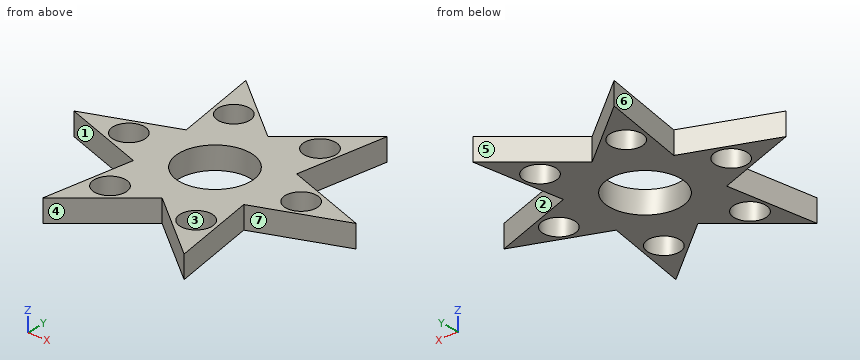
```python
from build123d import *

# Parameters (mm, degrees)
F0_R     = 4.9
F0_R_2   = 11.15
F1_DEPTH = 7


with BuildPart() as f1:
    # F0 (on Top) → F1 (new body)
    with BuildSketch(Plane.XY):
        Polygon((-7.7780097821, 13.4719081244), (0, 19.9143218109), (-22.0348406583, 38.1654635569), (-17.2463085873, 9.9571609054), align=None)
        with Locations((-13.4494397789, 23.2951130304)):
            Circle(F0_R, mode=Mode.SUBTRACT)
        with BuildLine():
            ThreePointArc((-6.4179147594, 13.9767918736), (0, 15.3798680403), (6.4179147594, 13.9767918736))
            Line((6.4179147594, 13.9767918736), (7.7780097821, 13.4719081244))
            Line((7.7780097821, 13.4719081244), (0, 19.9143218109))
            Line((0, 19.9143218109), (-7.7780097821, 13.4719081244))
            Line((-7.7780097821, 13.4719081244), (-6.4179147594, 13.9767918736))
        make_face()
        Polygon((0, 19.9143218109), (7.7780097821, 13.4719081244), (17.2463085873, 9.9571609054), (22.0348406583, 38.1654635569), align=None)
        with Locations((13.4494397789, 23.2951130304)):
            Circle(F0_R, mode=Mode.SUBTRACT)
        with BuildLine():
            ThreePointArc((8.8952994462, 12.5464731577), (13.3193564297, 7.6899340201), (15.3132142056, 1.4303187159))
            Line((15.3132142056, 1.4303187159), (15.5560195643, 0))
            Line((15.5560195643, 0), (17.2463085873, 9.9571609054))
            Line((17.2463085873, 9.9571609054), (7.7780097821, 13.4719081244))
            Line((7.7780097821, 13.4719081244), (8.8952994462, 12.5464731577))
        make_face()
        Polygon((17.2463085873, 9.9571609054), (15.5560195643, 0), (17.2463085873, -9.9571609054), (44.0696813166, 0), align=None)
        with Locations((26.8988795578, 0)):
            Circle(F0_R, mode=Mode.SUBTRACT)
        with BuildLine():
            ThreePointArc((15.3132142056, -1.4303187159), (15.3631955447, -0.7159354654), (15.3798680403, 0))
            ThreePointArc((15.3798680403, 0), (15.3631955447, 0.7159354654), (15.3132142056, 1.4303187159))
            ThreePointArc((15.3132142056, 1.4303187159), (13.3193564297, 7.6899340201), (8.8952994462, 12.5464731577))
            ThreePointArc((8.8952994462, 12.5464731577), (7.6899340201, 13.3193564297), (6.4179147594, 13.9767918736))
            ThreePointArc((6.4179147594, 13.9767918736), (0, 15.3798680403), (-6.4179147594, 13.9767918736))
            ThreePointArc((-6.4179147594, 13.9767918736), (-7.6899340201, 13.3193564297), (-8.8952994462, 12.5464731577))
            ThreePointArc((-8.8952994462, 12.5464731577), (-13.3193564297, 7.6899340201), (-15.3132142056, 1.4303187159))
            ThreePointArc((-15.3132142056, 1.4303187159), (-15.3798680403, 0), (-15.3132142056, -1.4303187159))
            ThreePointArc((-15.3132142056, -1.4303187159), (-13.3193564297, -7.6899340201), (-8.8952994462, -12.5464731577))
            ThreePointArc((-8.8952994462, -12.5464731577), (-7.6899340201, -13.3193564297), (-6.4179147594, -13.9767918736))
            ThreePointArc((-6.4179147594, -13.9767918736), (0, -15.3798680403), (6.4179147594, -13.9767918736))
            ThreePointArc((6.4179147594, -13.9767918736), (7.6899340201, -13.3193564297), (8.8952994462, -12.5464731577))
            ThreePointArc((8.8952994462, -12.5464731577), (13.3193564297, -7.6899340201), (15.3132142056, -1.4303187159))
        make_face()
        Circle(F0_R_2, mode=Mode.SUBTRACT)
        with BuildLine():
            Line((15.5560195643, 0), (15.3132142056, -1.4303187159))
            ThreePointArc((15.3132142056, -1.4303187159), (13.3193564297, -7.6899340201), (8.8952994462, -12.5464731577))
            Line((8.8952994462, -12.5464731577), (7.7780097821, -13.4719081244))
            Line((7.7780097821, -13.4719081244), (17.2463085873, -9.9571609054))
            Line((17.2463085873, -9.9571609054), (15.5560195643, 0))
        make_face()
        Polygon((22.0348406583, -38.1654635569), (17.2463085873, -9.9571609054), (7.7780097821, -13.4719081244), (0, -19.9143218109), align=None)
        with Locations((13.4494397789, -23.2951130304)):
            Circle(F0_R, mode=Mode.SUBTRACT)
        with BuildLine():
            Line((7.7780097821, -13.4719081244), (6.4179147594, -13.9767918736))
            ThreePointArc((6.4179147594, -13.9767918736), (0, -15.3798680403), (-6.4179147594, -13.9767918736))
            Line((-6.4179147594, -13.9767918736), (-7.7780097821, -13.4719081244))
            Line((-7.7780097821, -13.4719081244), (0, -19.9143218109))
            Line((0, -19.9143218109), (7.7780097821, -13.4719081244))
        make_face()
        Polygon((-22.0348406583, -38.1654635569), (0, -19.9143218109), (-7.7780097821, -13.4719081244), (-17.2463085873, -9.9571609054), align=None)
        with Locations((-13.4494397789, -23.2951130304)):
            Circle(F0_R, mode=Mode.SUBTRACT)
        with BuildLine():
            Line((-7.7780097821, -13.4719081244), (-8.8952994462, -12.5464731577))
            ThreePointArc((-8.8952994462, -12.5464731577), (-13.3193564297, -7.6899340201), (-15.3132142056, -1.4303187159))
            Line((-15.3132142056, -1.4303187159), (-15.5560195643, 0))
            Line((-15.5560195643, 0), (-17.2463085873, -9.9571609054))
            Line((-17.2463085873, -9.9571609054), (-7.7780097821, -13.4719081244))
        make_face()
        Polygon((-15.5560195643, 0), (-17.2463085873, 9.9571609054), (-44.0696813166, 0), (-17.2463085873, -9.9571609054), align=None)
        with Locations((-26.8988795578, 0)):
            Circle(F0_R, mode=Mode.SUBTRACT)
        with BuildLine():
            ThreePointArc((-15.3132142056, 1.4303187159), (-13.3193564297, 7.6899340201), (-8.8952994462, 12.5464731577))
            Line((-8.8952994462, 12.5464731577), (-7.7780097821, 13.4719081244))
            Line((-7.7780097821, 13.4719081244), (-17.2463085873, 9.9571609054))
            Line((-17.2463085873, 9.9571609054), (-15.5560195643, 0))
            Line((-15.5560195643, 0), (-15.3132142056, 1.4303187159))
        make_face()
        with BuildLine():
            ThreePointArc((6.4179147594, 13.9767918736), (7.6899340201, 13.3193564297), (8.8952994462, 12.5464731577))
            Line((8.8952994462, 12.5464731577), (7.7780097821, 13.4719081244))
            Line((7.7780097821, 13.4719081244), (6.4179147594, 13.9767918736))
        make_face()
        with BuildLine():
            ThreePointArc((-8.8952994462, 12.5464731577), (-7.6899340201, 13.3193564297), (-6.4179147594, 13.9767918736))
            Line((-6.4179147594, 13.9767918736), (-7.7780097821, 13.4719081244))
            Line((-7.7780097821, 13.4719081244), (-8.8952994462, 12.5464731577))
        make_face()
        with BuildLine():
            ThreePointArc((-15.3132142056, -1.4303187159), (-15.3798680403, 0), (-15.3132142056, 1.4303187159))
            Line((-15.3132142056, 1.4303187159), (-15.5560195643, 0))
            Line((-15.5560195643, 0), (-15.3132142056, -1.4303187159))
        make_face()
        with BuildLine():
            Line((-7.7780097821, -13.4719081244), (-6.4179147594, -13.9767918736))
            ThreePointArc((-6.4179147594, -13.9767918736), (-7.6899340201, -13.3193564297), (-8.8952994462, -12.5464731577))
            Line((-8.8952994462, -12.5464731577), (-7.7780097821, -13.4719081244))
        make_face()
        with BuildLine():
            Line((7.7780097821, -13.4719081244), (8.8952994462, -12.5464731577))
            ThreePointArc((8.8952994462, -12.5464731577), (7.6899340201, -13.3193564297), (6.4179147594, -13.9767918736))
            Line((6.4179147594, -13.9767918736), (7.7780097821, -13.4719081244))
        make_face()
        with BuildLine():
            ThreePointArc((15.3132142056, 1.4303187159), (15.3631955447, 0.7159354654), (15.3798680403, 0))
            ThreePointArc((15.3798680403, 0), (15.3631955447, -0.7159354654), (15.3132142056, -1.4303187159))
            Line((15.3132142056, -1.4303187159), (15.5560195643, 0))
            Line((15.5560195643, 0), (15.3132142056, 1.4303187159))
        make_face()
    extrude(amount=F1_DEPTH)


solid = f1.part
```
Source: CAD feature listing. Evaluate the final solid. Frame: model axes, mm. Face numbers are marked on the shaded views. A direction names the side the tool comes from. Coordinates: 2 decimals unless noted, no trailing zeros. Loops run counter-clockwise (first coordinate to the right, second up) from the corner with the lowest first, then second, coordinate; pieces in that order, holes last. Notation, with made-up numbers: (48.5, -32.5) -> (58.5, -32.5) arc R23 ccw to (58.5, -6.5) -> close; hole circle Ø6 at (63.5, 38). An arc over 180 degrees is marked (long way). One line per item, written item: value. Start each with the question number.
Q1. Set-up query: the marked faces 4, 5, 6 and 7. Return all of +Z, -Z, +X, -X, +Y, -Y with unobstructed straight access to the full face (end or side cutting, diameter ignored); none if empty.
Q2. Line query: line 1 along Y through (x, z) = (16, 6); line 2 along Y through (x, z) = (9.5, 5.25); line 3 along X through (y, z) = (-19.5, 1.75). Output: solid intervals per line, ascending.
Q3. Contact query for flat-ended pins moving along their axis: P1, Ø2, axis at y = 29, z = 5, coming from the -X side; P2, Ø9, axis at x = 26.9, y = 0, coming from the -Z side; P3, Ø1, axis at x = 12.5, z = 1, coming from the +Y side; P4, Ø1, axis at y = 28.5, z = 2, coming from the +X side. Output: stop coordinate, or through.
Q4. Mould query, pull axis X, two halves, no side actions, for the marked faces 1, 2 and 3. Classes: pulls with the +X half, pulls with the -X half, needs draft (parallel to the pull), parting line crosses it, or undercut.
Q5. Section query D-D, the plane y = -16.5. Return the cut outline in (x, z), and give its area (3 significant figures).
Q6. Section query C-C, the plane x = -33.5. Return the cut outline in (y, z), and give its area (3 significant figures).
Q7. Section query A-A, the plane z = 4.25. Return the cut outline in (x, y).
Q8. Section query B-B, the plane y = 25.5. Return the cut outline in (x, z), and give its area (3 significant figures).
Results:
1. face 4: +Z, -Z, -Y
1. face 5: +Z, -Z, +Y
1. face 6: +Z, -Z, -X
1. face 7: +Z, -Z, +X
2. line 1: -33.17 to -27.48, -19.11 to 19.11, 27.48 to 33.17
2. line 2: -27.78 to -26.2, -20.39 to -5.84, 5.84 to 20.39, 26.2 to 27.78
2. line 3: -18.87 to -16.55, -10.35 to 10.35, 16.55 to 18.87
3. P1: x = -20.65
3. P2: through
3. P3: y = 30.68
3. P4: x = 20.48
4. face 1: pulls with the -X half
4. face 2: pulls with the +X half
4. face 3: undercut
5. outline: (-18.36, 0) -> (18.36, 0) -> (18.36, 7) -> (-18.36, 7) -> close
5. area: 257 mm^2
6. outline: (-3.92, 0) -> (3.92, 0) -> (3.92, 7) -> (-3.92, 7) -> close
6. area: 54.9 mm^2
7. outline: (-44.07, 0) -> (-17.25, -9.96) -> (-22.03, -38.17) -> (0, -19.91) -> (22.03, -38.17) -> (17.25, -9.96) -> (44.07, 0) -> (17.25, 9.96) -> (22.03, 38.17) -> (0, 19.91) -> (-22.03, 38.17) -> (-17.25, 9.96) -> close; hole circle Ø9.8 at (-26.9, 0); hole circle Ø9.8 at (-13.45, -23.3); hole circle Ø9.8 at (-13.45, 23.3); hole circle Ø22.3 at (0, 0); hole circle Ø9.8 at (13.45, -23.3); hole circle Ø9.8 at (13.45, 23.3); hole circle Ø9.8 at (26.9, 0)
8. outline: (-19.88, 0) -> (-17.83, 0) -> (-17.83, 7) -> (-19.88, 7) -> close; (-9.07, 0) -> (-6.74, 0) -> (-6.74, 7) -> (-9.07, 7) -> close; (6.74, 0) -> (9.07, 0) -> (9.07, 7) -> (6.74, 7) -> close; (17.83, 0) -> (19.88, 0) -> (19.88, 7) -> (17.83, 7) -> close
8. area: 61.5 mm^2
